The model under review builds one solid part; all positions refer to its coordinate system, in mm. Face numbers are marked on the shaded views. A direction names the side the tool comes from. Coordinates: 2 decimals unless noted, no trailing zeros. Order: outer loops, then holes, each group sorted by start corner. A loop starts at its lowest first (then second) coordinate and runs counter-clockwise, first axis right, second up. Notation, with made-up numbers: (28, 57) -> (83, 57) arc R33 cw to (83, 89) -> close; hole circle Ø2 at (-2, -16.75). An arc over 180 degrees is marked (long way). Use one line per item in the form item = value. Start each with the question number.
(1) Mouldability with a two-part tool opening along Z and no side actions: class the marked faces 1, 2 and 3 as +Z half, -Z half, draft (parallel to the pull), parting line (faces both ways), or undercut.
(2) Take a section at D-D (z = 0). State the section outline as (x, y) points.
(3) Take a section at A-A (y = 14). State the section outline as (x, z) points, then the cut area to 3 significant figures.
(4) For the marked faces 4 and 5, list the 3-axis set-ups (+Z, -Z, +X, -X, +Y, -Y) from which the entire face can be reached by the end or side of a thin tool; tool diameter is ignored.
(5) Take a section at C-C (x = -34.5). State the section outline as (y, z) points, then the cut area to 3 significant figures.
(6) Insertion check: pin 1 Ø6 at (y, z) = (22, -4.5) entering from +X; pin 2 Ø1.4 at (x, y) = (57, 31) entering from -Z; pin 3 Ø8.5 at (y, z) = (23.5, -3) entering from +X. Each pin has a flat end and moves straight along its axis. Give the tip position at first contact, or say it passes through.
(7) Wall thickness on line 1 along X through (y, z) = (33, -9.5); line 2 along Z through (x, y) = (22, 37); line 3 along X through (y, z) = (16, -24): over which ranges is each line inside the solid? List them lowest first.
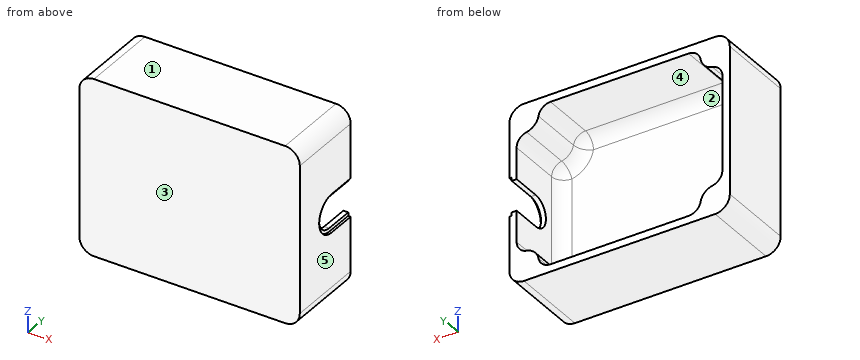
Autodesk Inventor part; units mm, degrees
ref_plane "YZ Plane" through (0, 0, 0) normal (1, 0, 0) x (0, 1, 0)
ref_plane "XZ Plane" through (0, 0, 0) normal (0, 1, 0) x (-1, 0, 0)
ref_plane "XY Plane" through (0, 0, 0) normal (0, 0, 1) x (1, 0, 0)
sketch "Sketch1" plane through (0, 0, 0) normal (0, 1, 0) x (-1, 0, 0)
  line L0 (57.15, 45.72) -> (-57.15, 45.72)
  line L1 (-57.15, 45.72) -> (-57.15, -45.72)
  line L2 (-57.15, -45.72) -> (57.15, -45.72)
  line L3 (57.15, -45.72) -> (57.15, 45.72)
  point P0 (0, 0)
  point P1 (-57.15, 0)
  point P2 (0, -45.72)
  dimension "d0" = 114.3
  dimension "d1" = 91.44
extrude "Extrusion1" add sketch "Sketch1" along normal blind 40.64
fillet "Fillet1" radius 7.62 4 edges at (-57.15, 20.32, 45.72) (57.15, 20.32, 45.72) (-57.15, 20.32, -45.72) (57.15, 20.32, -45.72)
sketch "Sketch2" plane through (0, 40.64, 0) normal (0, 1, 0) x (1, 0, 0)
  arc A0 (-57.15, -38.1) -> (-49.53, -45.72) centre (-49.53, -38.1) ccw
  line L0 (-57.15, 38.1) -> (-57.15, -38.1)
  circle A1 centre (-49.53, -38.1) radius 7.62
  arc A2 (-49.53, 45.72) -> (-57.15, 38.1) centre (-49.53, 38.1) ccw
  circle A3 centre (-49.53, 38.1) radius 7.62
  arc A4 (57.15, 38.1) -> (49.53, 45.72) centre (49.53, 38.1) ccw
  line L1 (49.53, 45.72) -> (-49.53, 45.72)
  circle A5 centre (49.53, 38.1) radius 7.62
  arc A6 (49.53, -45.72) -> (57.15, -38.1) centre (49.53, -38.1) ccw
  circle A7 centre (49.53, -38.1) radius 7.62
  line L2 (-53.34, -41.91) -> (53.34, -41.91)
  line L3 (53.34, -41.91) -> (53.34, 41.91)
  line L4 (53.34, 41.91) -> (-53.34, 41.91)
  line L5 (-53.34, 41.91) -> (-53.34, -41.91)
  point P0 (0, 0)
  point P1 (-53.34, 0)
  point P2 (0, 41.91)
  point P3 (-53.34, 31.5009)
  point P4 (-53.34, -31.5009)
  point P5 (-42.9309, -41.91)
  point P6 (42.9309, -41.91)
  point P7 (53.34, -31.5009)
  point P8 (53.34, 31.5009)
  point P9 (42.9309, 41.91)
  point P10 (-42.9309, 41.91)
  dimension "d5" = 3.81
  dimension "d6" = 3.81
extrude "Extrusion2" cut sketch "Sketch2" against normal blind 34.29 contours L5 A3 L4 A5 L3 A7 L2 A1
fillet "Fillet2" radius 6.35 16 edges at (-42.9309, 23.495, 41.91) (-53.34, 23.495, 31.5009) (0, 6.35, 41.91) (-53.34, 6.35, 0) (-53.34, 23.495, -31.5009) (-44.1418, 6.35, -32.7118) (-42.9309, 23.495, -41.91) (-44.1418, 6.35, 32.7118) (44.1418, 6.35, 32.7118) (42.9309, 23.495, 41.91) (53.34, 23.495, 31.5009) (53.34, 6.35, 0) (44.1418, 6.35, -32.7118) (53.34, 23.495, -31.5009) (42.9309, 23.495, -41.91) (0, 6.35, -41.91)
sketch "Sketch3" plane through (57.15, 0, 38.1) normal (1, 0, 0) x (0, 0, -1)
  line L0 (13.7372, 40.64) -> (62.4628, 40.64)
  line L1 (29.972, 40.64) -> (29.972, 25.4)
  arc A0 (29.972, 25.4) -> (46.228, 25.4) centre (38.1, 25.4) ccw
  line L2 (46.228, 25.4) -> (46.228, 40.64)
  line L3 (28.194, 40.64) -> (28.194, 25.4)
  arc A1 (28.194, 25.4) -> (48.006, 25.4) centre (38.1, 25.4) ccw
  line L4 (48.006, 25.4) -> (48.006, 40.64)
  point P0 (38.1, 0)
  point P1 (38.1, 40.64)
  point P2 (28.194, 40.64)
  dimension "d10" = 15.24
  dimension "d11" = 8.128
  dimension "d12" = 1.778
extrude "Extrusion3" cut sketch "Sketch3" against normal up to surface (3.81 mm away) contours L0 L2 A0 L1
extrude "Extrusion4" cut sketch "Sketch3" against normal blind 1.27 contours L0 L1 A0 L2 L4 A1 L3
equation "\"d6\" = d5"
properties part number "Machined Base" material "Steel, Mild"
Findings:
q1.face_1 = +Z half
q1.face_2 = undercut
q1.face_3 = draft
q2.outline = (-57.15, 0) -> (57.15, 0) -> (57.15, 15.49) -> (55.88, 15.49) -> (55.88, 17.27) -> (53.34, 17.27) -> (53.34, 12.7) arc R6.35 cw to (46.99, 6.35) -> (-46.99, 6.35) arc R6.35 cw to (-53.34, 12.7) -> (-53.34, 40.64) -> (-57.15, 40.64) -> close
q3.outline = (-57.15, -38.1) arc R7.62 ccw to (-49.53, -45.72) -> (49.53, -45.72) arc R7.62 ccw to (57.15, -38.1) -> (57.15, 38.1) arc R7.62 ccw to (49.53, 45.72) -> (-49.53, 45.72) arc R7.62 ccw to (-57.15, 38.1) -> close; hole (-53.34, -24.36) arc R6.35 ccw to (-48.14, -30.61) arc R7.62 cw to (-42.04, -36.71) arc R6.35 ccw to (-35.79, -41.91) -> (35.79, -41.91) arc R6.35 ccw to (42.04, -36.71) arc R7.62 cw to (48.14, -30.61) arc R6.35 ccw to (53.34, -24.36) -> (53.34, 24.36) arc R6.35 ccw to (48.14, 30.61) arc R7.62 cw to (42.04, 36.71) arc R6.35 ccw to (35.79, 41.91) -> (-35.79, 41.91) arc R6.35 ccw to (-42.04, 36.71) arc R7.62 cw to (-48.14, 30.61) arc R6.35 ccw to (-53.34, 24.36) -> close
q3.area = 1,990 mm²
q4.face_4 = +Y
q4.face_5 = +Z, -Z, +X, +Y, -Y
q5.outline = (0, -45.72) -> (40.64, -45.72) -> (40.64, -41.91) -> (12.7, -41.91) arc R6.35 cw to (6.35, -35.56) -> (6.35, 35.56) arc R6.35 cw to (12.7, 41.91) -> (40.64, 41.91) -> (40.64, 45.72) -> (0, 45.72) -> close
q5.area = 859 mm²
q6.pin_1 = 55.88
q6.pin_2 = -41.6
q6.pin_3 = -53.34
q7.line_1 = -57.15 to -53.34, 53.34 to 55.88
q7.line_2 = -45.72 to -41.91, 41.91 to 45.72
q7.line_3 = -57.15 to -53.34, 53.34 to 57.15
